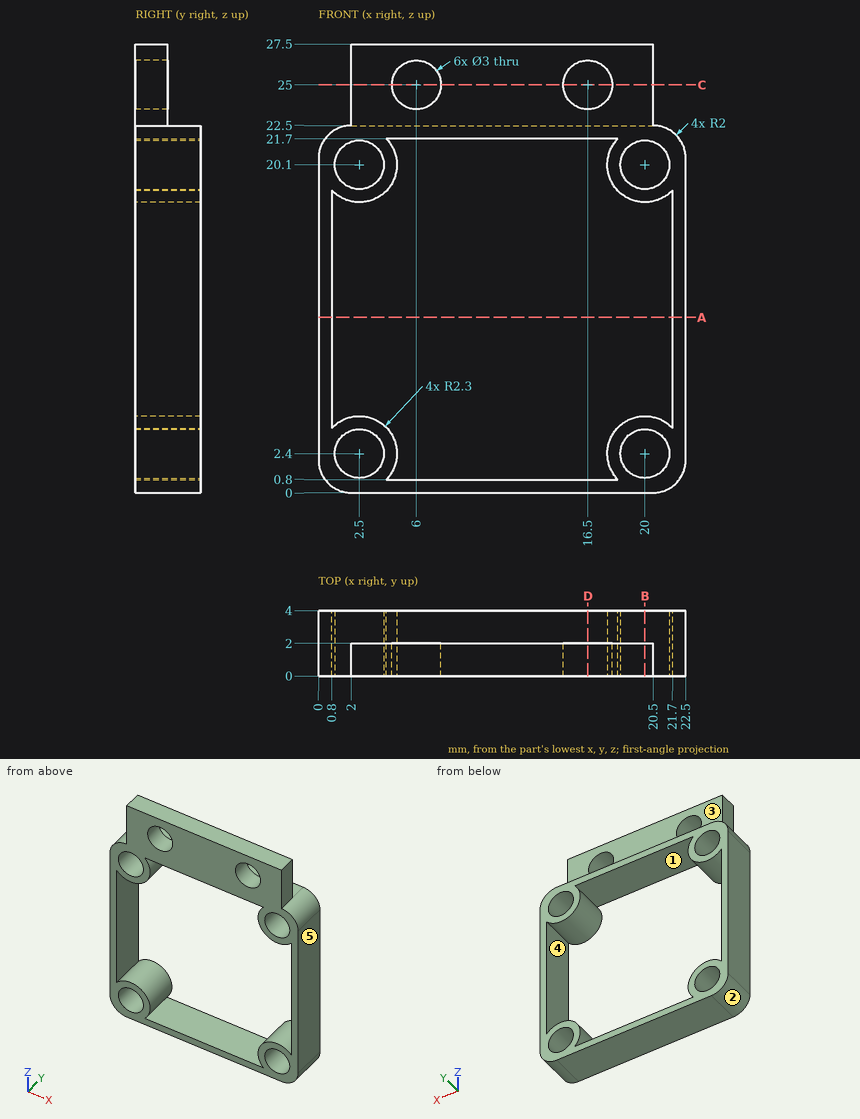
Print and shaded views of the part. All mm, measured from the part's lowest x, y and z. A direction names the side the tool comes from. Give positions to 0.01 mm unless a question says otherwise; leave off trailing zeros. Loops run counter-clockwise (first coordinate to the right, second up) from the corner with the lowest first, then second, coordinate; pieces in that order, holes last. Notation, with made-up numbers: (-35, 15) - (-12, 15) arc R21 ccw to (-12, 22) - close; hole circle Ø11 at (64, 47.5). An arc over 180 degrees is marked (long way). Use a Markdown table: item, result.
(1) Pull direction X, two halves, no side cores. Call the marked faces 3, 4 and 5: +X half, -X half, draft (parallel to the pull), parting line (faces both ways), or undercut.
Taken from the geometry:
| item | result |
|---|---|
| face 3 | draft |
| face 4 | undercut |
| face 5 | +X half |
(2) Band-saw the part on C-C (z = 25). Give the cut face in (x, y).
Taken from the geometry:
| item | result |
|---|---|
| outline | (2, 0) - (4.5, 0) - (4.5, 2) - (2, 2) - close; (7.5, 0) - (15, 0) - (15, 2) - (7.5, 2) - close; (18, 0) - (20.5, 0) - (20.5, 2) - (18, 2) - close |
(3) Wall check: line 1 along X through (y, z) = (0.55, 25); line 2 along Z through (x, y) = (6, 1.65); line 3 along Z through (x, y) = (13, 2.55). Give the ranges that are in metal, low to high.
Taken from the geometry:
| item | result |
|---|---|
| line 1 | 2 to 4.5, 7.5 to 15, 18 to 20.5 |
| line 2 | 0 to 0.8, 21.7 to 23.5, 26.5 to 27.5 |
| line 3 | 0 to 0.8, 21.7 to 22.5 |
(4) Drop flat-ended pins along their axis: pin 1 Ø1.6 at (y, z) = (1, 25.5) entering from +X; pin 2 Ø1 at (y, z) = (1.5, 24.5) entering from -X; pin 3 Ø2.5 at (x, z) = (2.5, 2.4) entering from +Y. Give the stop position or say it passes through.
Taken from the geometry:
| item | result |
|---|---|
| pin 1 | x = 20.5 |
| pin 2 | x = 2 |
| pin 3 | through |
(5) Band-saw the part on B-B (x = 20). Give the cut face in (y, z), and give its area (3 significant figures).
Taken from the geometry:
| item | result |
|---|---|
| outline | (0, 0) - (4, 0) - (4, 0.9) - (0, 0.9) - close; (0, 3.9) - (4, 3.9) - (4, 4.7) - (0, 4.7) - close; (0, 17.8) - (4, 17.8) - (4, 18.6) - (0, 18.6) - close; (0, 21.6) - (4, 21.6) - (4, 22.5) - (2, 22.5) - (2, 27.5) - (0, 27.5) - close |
| area | 23.6 mm2 |
(6) Band-saw the part on A-A (z = 10.75). Give the cut face in (x, y), and give its area (3 significant figures).
Taken from the geometry:
| item | result |
|---|---|
| outline | (0, 0) - (0.8, 0) - (0.8, 4) - (0, 4) - close; (21.7, 0) - (22.5, 0) - (22.5, 4) - (21.7, 4) - close |
| area | 6.40 mm2 |
(7) Which spindle directions (+Z, -Z, +X, -X, +Y, -Y) get a long thin tool onto all of the face, cutting with end or side? Do the marked faces 1 and 2. Say none if no direction does.
Taken from the geometry:
| item | result |
|---|---|
| face 1 | +Y, -Y |
| face 2 | -Z, -X, +Y, -Y |
(8) Band-saw the part on D-D (x = 16.5). Give the cut face in (y, z), and give its area (3 significant figures).
Taken from the geometry:
| item | result |
|---|---|
| outline | (0, 0) - (4, 0) - (4, 0.8) - (0, 0.8) - close; (0, 21.7) - (4, 21.7) - (4, 22.5) - (2, 22.5) - (2, 23.5) - (0, 23.5) - close; (0, 26.5) - (2, 26.5) - (2, 27.5) - (0, 27.5) - close |
| area | 10.4 mm2 |
